```python
from build123d import *


with BuildPart() as f1:
    # F0 (on Front) → F1 (revolve)
    with BuildSketch(Plane.XZ):
        with BuildLine():
            Line((-13.25, 755), (-13.25, 740))
            Line((-13.25, 740), (-18.75, 740))
            Line((-18.75, 740), (-18.75, 86))
            ThreePointArc((-18.75, 86), (-18.457107, 85.292893), (-17.75, 85))
            Line((-17.75, 85), (-15.75, 85))
            Line((-15.75, 85), (-4.238613, 1.726134))
            ThreePointArc((-4.238613, 1.726134), (-3.571276, 0.492066), (-2.257452, 0))
            Line((-2.257452, 0), (0, 0))
            Line((0, 0), (0, 634))
            Line((0, 634), (-6.5, 634))
            Line((-6.5, 634), (-6.5, 755))
            Line((-6.5, 755), (-13.25, 755))
        make_face()
    revolve(axis=Axis((0, 0, 317), (0, 0, -1)))


solid = f1.part
```
The model under review builds one solid part; all positions refer to its coordinate system, in mm. A direction names the side the tool comes from. Give positions to 0.01 mm unless a question says otherwise; leave off trailing zeros. Loops run counter-clockwise (first coordinate to the right, second up) from the corner with the lowest first, then second, coordinate; pieces in that order, holes last. Notation, with made-up numbers: (54, 68.25) -> (71, 68.25) arc R21 ccw to (71, 83.25) -> close; hole circle Ø11 at (-6, 23.25). An arc over 180 degrees is marked (long way). Use CSV: the item, a comma, the result in double quotes.
1. To check wall thickness, follow probe 1 along Y at (x, z) = (0, 725); probe 2 along Z at (x, y) = (16, 1); probe 3 along Y at (x, z) = (-2, 204). State the ranges of each line that lie inside material, in increasing order. Write a range as from..to.
Result:
probe 1,"y = -18.75..-6.5, 6.5..18.75"
probe 2,"z = 85..740"
probe 3,"y = -18.64..18.64"
2. The part is to be moulded in two halves that separate along Y. For faces 1 (the face through (-7.123, 11.172, 747.395)), 2 (the face through (5.158, -3.955, 695.347)), 3 (the face through (0, 0, 634)), 4 (the face through (6, 3, 755)), say which applies: +Y half, -Y half, draft (parallel to the pull), parting line (faces both ways), or undercut.
Result:
face 1,"parting line"
face 2,"undercut"
face 3,"undercut"
face 4,"draft"
3. Consider section A-A, the plane z = 550.5. Write out the cut boundary in (x, y), then the cut area to 3 significant figures.
Result:
outline,"circle Ø37.5 at (0, 0)"
area,"1,100 mm²"
4. Machinability: for faces 5 (the face through (2.44, 18.59, 408.42)), 6 (the face through (-13, -4, 740)), 7 (the face through (11, -12, 85)), which of the approach directions +Z, -Z, +X, -X, +Y, -Y give a long, thin tool a straight path to every point of the face, cutting with its end or side? Answer none if there is none.
Result:
face 5,"+Z, -Z"
face 6,"+Z"
face 7,"-Z"
5. For P1, Ø5, axis at x = -2.5, z = 678.5, coming from the +Y side; P2, Ø1, axis at x = -14, y = -14.5, coming from the -Z side; P3, Ø11.5, axis at x = 0, y = 0, coming from the +Z side; P4, Ø4, axis at x = -12, z = 674.5, coming from the -Y side, all flat-tipped, find the tip position at first contact; note any pin that passes through.
Result:
P1,"stops at y = 18.75"
P2,"passes through"
P3,"stops at z = 634"
P4,"stops at y = -15.86"
